For this review, use the dimensioned drawing (mm, ordinates from the lowest corner) and the shaded views. A direction names the side the tool comes from. Coordinates: 2 decimals unless noted, no trailing zeros. Loops run counter-clockwise (first coordinate to the right, second up) from the corner with the lowest first, then second, coordinate; pieces in that order, holes last. Notation, with made-up numbers: M -38,42.25 L -17,42.25 A16 cw -17,55.25 Z; hole C 7.25,11.5 d10. An arc over 180 degrees is marked long. One line per item, written item: value.
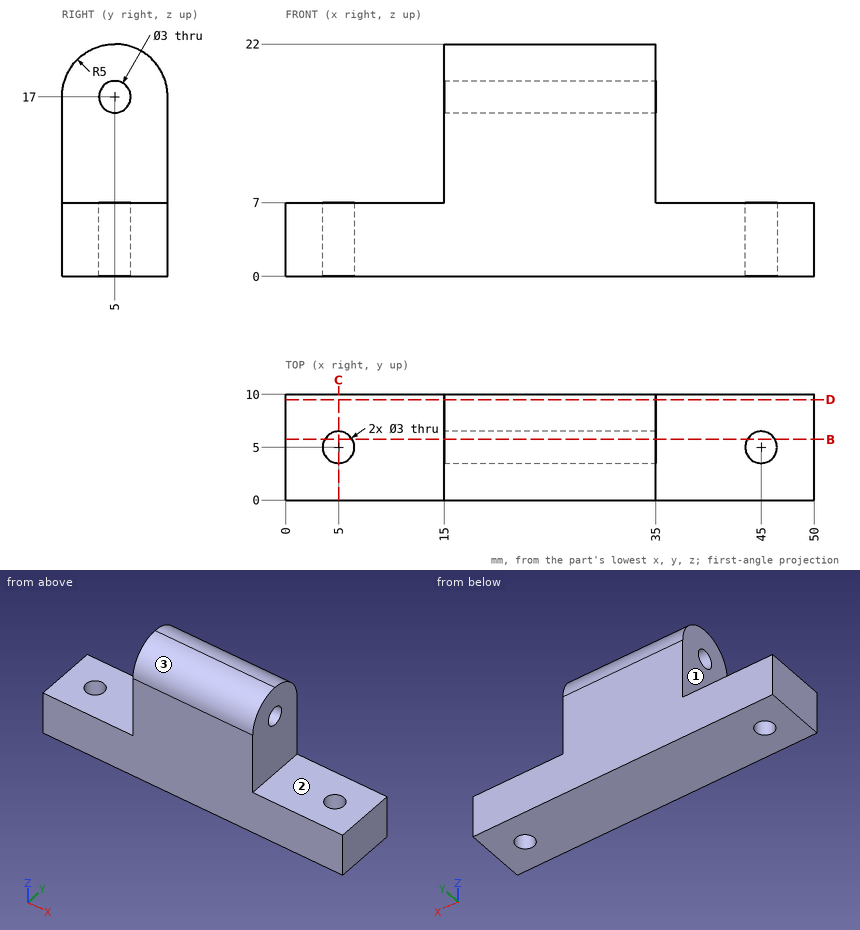
(1) We need section D-D on y = 9.5. State the section outline as (x, z) points.
Reply:
outline: M 0,0 L 50,0 L 50,7 L 35,7 L 35,19.18 L 15,19.18 L 15,7 L 0,7 Z
(2) We need section B-B on y = 5.75. State the section outline as (x, z) points.
Reply:
outline: M 0,0 L 3.7,0 L 3.7,7 L 0,7 Z; M 6.3,0 L 43.7,0 L 43.7,7 L 35,7 L 35,15.7 L 15,15.7 L 15,7 L 6.3,7 Z; M 15,18.3 L 35,18.3 L 35,21.94 L 15,21.94 Z; M 46.3,0 L 50,0 L 50,7 L 46.3,7 Z
(3) Tool access review of the marked faces 1, 2 and 3: name each direction out of +Z, -Z, +X, -X, +Y, -Y from which nothing blocks a thin tool from reaching the whole face with its end or side.
Reply:
face 1: +Z, -X, +Y, -Y
face 2: +Z, +X, +Y, -Y
face 3: +Z, +X, -X, -Y
(4) To check wall thickness, follow line 1 along Y through (x, z) = (5, 4); line 2 along Z through (x, y) = (4, 2.5); line 3 along X through (y, z) = (3.75, 12.75). State the ranges of each line that lie inside material, in increasing order. Write a range as [from, to].
Reply:
line 1: y = [0, 3.5], [6.5, 10]
line 2: z = [0, 7]
line 3: x = [15, 35]
(5) Insertion check: pin 1 (5 mm diameter, centred on y = 4, z = 13.5, fed in from +X); pin 2 (5 mm diameter, centred on y = 6, z = 6.5, fed in from -X); pin 3 (4 mm diameter, centred on y = 5, z = 17, fed in from -X); pin 4 (5 mm diameter, centred on x = 6.5, y = 6.5, fed in from +Z). Each pin has a flat end and moves straight along its axis. Give the tip position at first contact, or say it passes through.
Reply:
pin 1: stops at x = 35
pin 2: stops at x = 0
pin 3: stops at x = 15
pin 4: stops at z = 7
(6) We need section C-C on x = 5. State the section outline as (y, z) points, then the cut area to 3 significant figures.
Reply:
outline: M 0,0 L 3.5,0 L 3.5,7 L 0,7 Z; M 6.5,0 L 10,0 L 10,7 L 6.5,7 Z
area: 49.0 mm2
